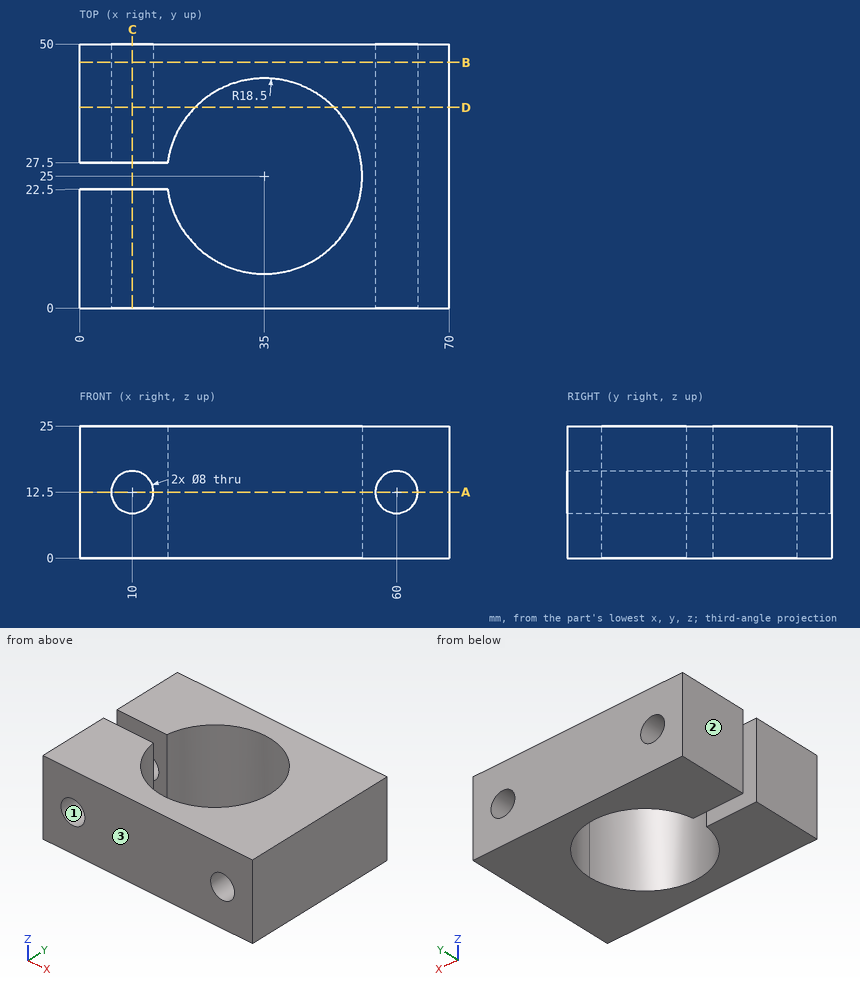
The figure shows three views and two pictorial views of one solid part (mm, origin at its lowest corner). Answer the questions. Round coordinates to 2 decimals unless told otherwise and drop trailing zeros. Write each loop counter-clockwise with the first axis right and the second up, starting at its lowest first coordinate (ties: lowest second). Pieces come first, ordered by that corner, then holes. Notation, with made-up numbers: (-9.75, 4.5) -> (34.25, 4.5) arc R19 ccw to (34.25, 41.5) -> close; hole circle Ø9 at (59.5, 69.5). An arc over 180 degrees is marked (long way). Answer as a JSON object with one key per item and string values. Group by question number.
Q1. Section A-A (z = 12.5) is taken. Write down the section's boundary in (x, y), plus the area to 3 significant figures.
Q2. Section C-C (x = 10) is taken. Write down the section's boundary in (y, z), plus the area to 3 significant figures.
Q3. Section D-D (y = 38) is taken. Write down the section's boundary in (x, z).
Q4. Determine the mould class of the marked faces 1, 2 and 3 for opening direction X: pulls with the +X half, pulls with the -X half, needs draft (parallel to the pull), parting line crosses it, or undercut.
Q5. Straight lines are drawn through the part: line 1 along X through (y, z) = (45.25, 12.5); line 2 along X through (y, z) = (30, 11); line 3 along Y through (x, z) = (3.5, 13.5). For each, find the intervals that lie inside material, in ascending order.
Q6. Section B-B (y = 46.5) is taken. Write down the section's boundary in (x, z).
Check values:
{
 "1": {"outline": "(0, 0) -> (6, 0) -> (6, 22.5) -> (0, 22.5) -> close; (0, 27.5) -> (6, 27.5) -> (6, 50) -> (0, 50) -> close; (14, 0) -> (56, 0) -> (56, 50) -> (14, 50) -> (14, 27.5) -> (16.67, 27.5) arc R18.5 cw (long way) to (16.67, 22.5) -> (14, 22.5) -> close; (64, 0) -> (70, 0) -> (70, 50) -> (64, 50) -> close", "area": "1,580 mm^2"},
 "2": {"outline": "(0, 0) -> (22.5, 0) -> (22.5, 8.5) -> (0, 8.5) -> close; (0, 16.5) -> (22.5, 16.5) -> (22.5, 25) -> (0, 25) -> close; (27.5, 0) -> (50, 0) -> (50, 8.5) -> (27.5, 8.5) -> close; (27.5, 16.5) -> (50, 16.5) -> (50, 25) -> (27.5, 25) -> close", "area": "765 mm^2"},
 "3": {"outline": "(0, 0) -> (21.84, 0) -> (21.84, 25) -> (0, 25) -> close; (48.16, 0) -> (70, 0) -> (70, 25) -> (48.16, 25) -> close; hole circle Ø8 at (10, 12.5); hole circle Ø8 at (60, 12.5)"},
 "4": {"face 1": "undercut", "face 2": "pulls with the -X half", "face 3": "needs draft"},
 "5": {"line 1": "0 to 6, 14 to 56, 64 to 70", "line 2": "0 to 6.29, 13.71 to 17.19, 52.81 to 56.29, 63.71 to 70", "line 3": "0 to 22.5, 27.5 to 50"},
 "6": {"outline": "(0, 0) -> (70, 0) -> (70, 25) -> (0, 25) -> close; hole circle Ø8 at (10, 12.5); hole circle Ø8 at (60, 12.5)"}
}
